Autodesk Inventor part; units mm, degrees
ref_plane "YZ Plane" through (0, 0, 0) normal (1, 0, 0) x (0, 1, 0)
ref_plane "XZ Plane" through (0, 0, 0) normal (0, 1, 0) x (-1, 0, 0)
ref_plane "XY Plane" through (0, 0, 0) normal (0, 0, 1) x (1, 0, 0)
sketch "Sketch1" plane through (0, 0, 0) normal (0, 0, 1) x (1, 0, 0)
  circle A0 centre (0, 0) radius 18
  circle A1 centre (0, 7.12) radius 6
  line L0 (0, 0) -> (0, 7.12) construction
  dimension "d0" = 36
  dimension "d1" = 12
  dimension "d2" = 7.12
extrude "Extrusion1" add sketch "Sketch1" along normal mid plane 5
sketch "Sketch2" plane through (0, 0, -2.5) normal (0, 0, -1) x (-1, 0, 0)
  circle A0 centre (0, 0) radius 15.425 construction
  circle A1 centre (0, 7.12) radius 6 construction
  line L0 (0, 7.12) -> (0, 7.7125) construction
  point P0 (0, -15.425)
  point P1 (13.3584, 7.7125)
  point P2 (-13.3584, 7.7125)
  dimension "d11" = 360
hole "Hole1" at (0, -15.425, -2.5) at (-13.3584, 7.7125, -2.5) at (13.3584, 7.7125, -2.5) direction (0, 0, 1) diameter 2.4 end through all counterbore diameter 4.4 counterbore depth 3
sketch "Sketch3" plane through (0, 0, -2.5) normal (0, 0, -1) x (-1, 0, 0)
  circle A0 centre (-13.3584, 7.7125) radius 2.2 construction
  circle A1 centre (-13.3584, 7.7125) radius 1.2 construction
  line L0 (-13.3584, 7.7125) -> (0, 0) construction
  line L1 (0, 0) -> (-9.6467, 13.7769) construction
  circle A2 centre (0, 0) radius 15.425 construction
  circle A3 centre (0, 7.12) radius 6 construction
  line L2 (0, 0) -> (0, 7.12) construction
  point P0 (-8.6036, 12.2873)
  dimension "d37" = 30.85
  dimension "d20" = 25
  dimension "d21" = 15
  dimension "d38" = 60
  dimension "d39" = 7.12
hole "Hole2" at (8.6036, 12.2873, -2.5) direction (0, 0, 1) diameter 2.459 end through all
pattern_circular "Circular Pattern1" count 3 over 360 about axis through (0, 0, 0) along (0, 0, 1) of "Hole2"
properties part number "P21" material "Aluminium"
Work out the finished part from the listing and answer in its coordinate system (mm). A direction names the side the tool comes from. Round coordinates to 2 decimals unless told otherwise and drop trailing zeros. Write each loop counter-clockwise with the first axis right and the second up, starting at its lowest first coordinate (ties: lowest second). Pieces come first, ordered by that corner, then holes.
1) A cutting plane is placed at A-A on x = 0. Determine the outline of the cut face in (y, z) (3 decimals).
2) Determine the mould class of faces 1 (the face through (-2.343, -17.847, -0.035)), 2 (the face through (0, 0, -2.5)), 3 (the face through (13.306, 6.514, 1.514)) for opening direction X: pulls with the +X half, pulls with the -X half, needs draft (parallel to the pull), parting line crosses it, or undercut.
3) Consider probe 1 along Y at (x, z) = (0, 1.1) (3 decimals); probe 2 along Y at (x, z) = (-14, -2.05); probe 3 along X at (y, z) = (8, -2.1). Determine where each line is inside the solid, lowest interval first.
4) Flat-ended cylindrical pins translate along their axes: P1, Ø1.5, axis at y = -6, z = -1.5, coming from the -X side; P2, Ø2, axis at x = -13.5, y = 7, coming from the -Z side; P3, Ø2, axis at y = 6, z = 0, coming from the -X side. Find the tip coordinate at first contact, or state that the pin passes through.
5) A cutting plane is placed at C-C on y = 7.12. Determine the outline of the cut face in (x, z), and give its area (3 significant figures).
6) Which of the six approach directions +Z, -Z, +X, -X, +Y, -Y give full straight-line access (tool end or side, diameter ignored) to faces 4 (the face through (-0.053, -16.624, 1.514)), 5 (the face through (0.84, -13.39, -0.98))?
7) A cutting plane is placed at B-B on x = -4.5. Determine the outline of the cut face in (y, z).
8) A cutting plane is placed at D-D on z = -0.8. Determine the outline of the cut face in (x, y) (1 decimal), and give its area (3 significant figures).
Entries:
1. outline: (-18, -2.5) - (-17.625, -2.5) - (-17.625, 0.5) - (-16.625, 0.5) - (-16.625, 2.5) - (-18, 2.5) - close; (-14.225, 0.5) - (-13.225, 0.5) - (-13.225, -2.5) - (1.12, -2.5) - (1.12, 2.5) - (-14.225, 2.5) - close; (13.12, -2.5) - (18, -2.5) - (18, 2.5) - (13.12, 2.5) - close
2. face 1: parting line crosses it
2. face 2: needs draft
2. face 3: undercut
3. probe 1: y = -18 to -16.625, -14.225 to 1.12, 13.12 to 18
3. probe 2: y = -11.31 to 0.52, 2.1 to 5.61, 9.82 to 11.31
3. probe 3: x = -16.12 to -15.54, -11.18 to -5.94, 5.94 to 11.18, 15.54 to 16.12
4. P1: stops at x = -17.22
4. P2: stops at z = 0.5
4. P3: stops at x = -17.29
5. outline: (-16.53, -2.5) - (-15.48, -2.5) - (-15.48, 0.5) - (-14.4, 0.5) - (-14.4, 2.5) - (-16.53, 2.5) - close; (-12.31, 0.5) - (-11.24, 0.5) - (-11.24, -2.5) - (-6, -2.5) - (-6, 2.5) - (-12.31, 2.5) - close; (6, -2.5) - (11.24, -2.5) - (11.24, 0.5) - (12.31, 0.5) - (12.31, 2.5) - (6, 2.5) - close; (14.4, 0.5) - (15.48, 0.5) - (15.48, -2.5) - (16.53, -2.5) - (16.53, 2.5) - (14.4, 2.5) - close
5. area: 71.5 mm2
6. face 4: +Z, -Z
6. face 5: -Z
7. outline: (-17.43, -2.5) - (3.15, -2.5) - (3.15, 2.5) - (-17.43, 2.5) - close; (11.09, -2.5) - (17.43, -2.5) - (17.43, 2.5) - (11.09, 2.5) - close
8. outline: circle Ø36 at (0, 0); hole circle Ø2.5 at (-14.9, 1.3); hole circle Ø4.4 at (-13.4, 7.7); hole circle Ø12 at (0, 7.1); hole circle Ø4.4 at (0, -15.4); hole circle Ø2.5 at (6.3, -13.6); hole circle Ø2.5 at (8.6, 12.3); hole circle Ø4.4 at (13.4, 7.7)
8. area: 845 mm2
